Design review of the part built by this model. Coordinates are the model's own, in mm. Face numbers are marked on the shaded views. A direction names the side the tool comes from. Coordinates: 2 decimals unless noted, no trailing zeros. Write each loop counter-clockwise with the first axis right and the second up, starting at its lowest first coordinate (ties: lowest second). Pieces come first, ordered by that corner, then holes. Notation, with made-up numbers: (17, -1.75) - (26, -1.75) arc R22 cw to (26, 16.25) - close; hole circle Ø1 at (-1, 64). An arc over 180 degrees is marked (long way). One line per item, written item: value.
from build123d import *

# Parameters (mm, degrees)
SKETCH1_W                  = 60
SKETCH1_H                  = 45
BOSS_EXTRUDE1_DEPTH        = 11
SKETCH3_W                  = 44
SKETCH3_H                  = 11
FAN_DEPTH                  = 42
SKETCH4_R                  = 1.25
SCREWS_DEPTH               = 10
F_3_4_3_4_DIAMETER_HOLE1_D = 3.4


with BuildPart() as part:
    # Sketch1 → Boss-Extrude1 (new body)
    with BuildSketch(Plane.XY):
        with Locations((30, 22.5)):
            Rectangle(SKETCH1_W, SKETCH1_H)
    extrude(amount=BOSS_EXTRUDE1_DEPTH)

    # Sketch3 → fan (cut)
    with BuildSketch(Plane(origin=(0, 45, 0), x_dir=(1, 0, 0), z_dir=(0, 1, 0))):
        with Locations((30, -5.5)):
            Rectangle(SKETCH3_W, SKETCH3_H)
    extrude(amount=-FAN_DEPTH, mode=Mode.SUBTRACT)

    # Sketch4 → screws (cut)
    with BuildSketch(Plane(origin=(0, 45, 0), x_dir=(1, 0, 0), z_dir=(0, 1, 0))):
        with Locations(Location((5, -4, 0), (0, 0, 270))):
            Circle(SKETCH4_R)
        with Locations(Location((55, -4, 0), (0, 0, 270))):
            Circle(SKETCH4_R)
    extrude(amount=-SCREWS_DEPTH, mode=Mode.SUBTRACT)

    # Ø3.4 (3.4) Diameter Hole1 (through all)
    with Locations(Plane(origin=(0, 0, 0), x_dir=(-1, 0, 0), z_dir=(0, 0, -1))):
        with Locations((-4, 30), (-4, 10), (-56, 10), (-56, 30)):
            Hole(F_3_4_3_4_DIAMETER_HOLE1_D / 2)


solid = part.part
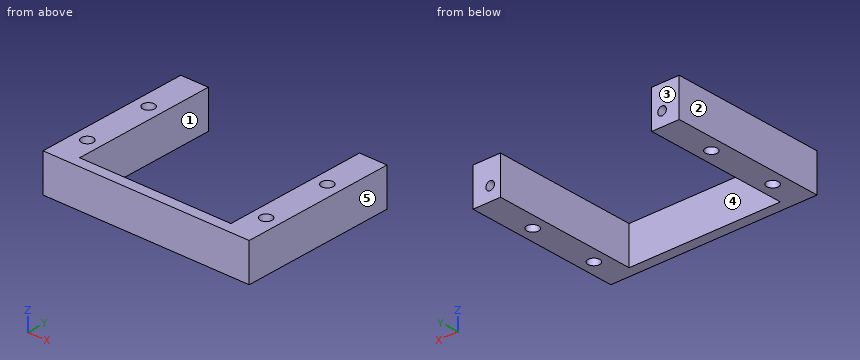
1. Consider section C-C, the plane y = 11. Write out the cut boundary in (x, z), then the cut area to 3 significant figures.
Answer block:
outline: (0, 0) - (2.63, 0) - (2.63, 11) - (0, 11) - close; (5.37, 0) - (8, 0) - (8, 11) - (5.37, 11) - close; (52, 0) - (54.63, 0) - (54.63, 11) - (52, 11) - close; (57.37, 0) - (60, 0) - (60, 11) - (57.37, 11) - close
area: 116 mm^2
2. For the marked faces 4 and 5, list the 3-axis set-ups (+Z, -Z, +X, -X, +Y, -Y) from which the entire face can be reached by the end or side of a thin tool; tool diameter is ignored.
Answer block:
face 4: +Z, -Z, +Y
face 5: +Z, -Z, +X, +Y, -Y
3. Mouldability with a two-part tool opening along X and no side actions: class the marked faces 1, 2 and 3 as released by +X, released by -X, zero draft, split by the parting line, or undercut.
Answer block:
face 1: undercut
face 2: released by -X
face 3: zero draft
4. Consider section B-B, the plane z = 4. Write out the cut boundary in (x, y).
Answer block:
outline: (0, 0) - (60, 0) - (60, 45) - (56.25, 45) - (56.25, 35) - (53.75, 35) - (53.75, 45) - (52, 45) - (52, 3) - (8, 3) - (8, 45) - (6.25, 45) - (6.25, 35) - (3.75, 35) - (3.75, 45) - (0, 45) - close; hole circle Ø3.4 at (4, 10); hole circle Ø3.4 at (4, 30); hole circle Ø3.4 at (56, 10); hole circle Ø3.4 at (56, 30)
5. Insertion check: pin 1 Ø2 at (x, y) = (4, 10) entering from -Z; pin 2 Ø1.2 at (x, z) = (5, 4) entering from +Y; pin 3 Ø1.5 at (x, z) = (16, 6.5) entering from +Y. Each pin has a flat end and moves straight along its axis. Give the tip position at first contact, or say it passes through.
Answer block:
pin 1: passes through
pin 2: stops at y = 35
pin 3: stops at y = 3
6. Wall thickness on line 1 along Y through (x, z) = (56, 3.5); line 2 along X through (y, z) = (26.5, 3); line 3 along X through (y, z) = (39.5, 4): over which ranges is each line inside the solid? List them lowest first.
Answer block:
line 1: y = 0 to 8.3, 11.7 to 28.3, 31.7 to 35
line 2: x = 0 to 8, 52 to 60
line 3: x = 0 to 3.75, 6.25 to 8, 52 to 53.75, 56.25 to 60
7. Consider section A-A, the plane y = 27. Write out the cut boundary in (x, z), then the cut area to 3 significant figures.
Answer block:
outline: (0, 0) - (8, 0) - (8, 11) - (0, 11) - close; (52, 0) - (60, 0) - (60, 11) - (52, 11) - close
area: 176 mm^2
8. Consider section D-D, the plane x = 55. Write out the cut boundary in (y, z), then the cut area to 3 significant figures.
Answer block:
outline: (0, 0) - (8.63, 0) - (8.63, 11) - (0, 11) - close; (11.37, 0) - (28.63, 0) - (28.63, 11) - (11.37, 11) - close; (31.37, 0) - (45, 0) - (45, 2.75) - (35, 2.75) - (35, 5.25) - (45, 5.25) - (45, 11) - (31.37, 11) - close
area: 410 mm^2
